from build123d import *

# Parameters (mm, degrees)
SKETCH1_R           = 2.5
BOSS_EXTRUDE1_DEPTH = 30
SKETCH6_R           = 3.75
BOSS_EXTRUDE6_DEPTH = 15
BOSS_EXTRUDE2_DEPTH = 2.5
SKETCH3_R           = 2.5
BOSS_EXTRUDE3_DEPTH = 2.8
BOSS_EXTRUDE4_START = 2.8
BOSS_EXTRUDE4_DEPTH = 2.8
SKETCH5_R           = 2.5
BOSS_EXTRUDE5_DEPTH = 2.8


with BuildPart() as part:
    # Sketch1 → Boss-Extrude1 (new, symmetric)
    with BuildSketch(Plane(origin=(0, 0, 0), x_dir=(1, 0, 0), z_dir=(0, 1, 0))):
        with Locations(Location((0, 0, 0), (0, 0, 270))):
            Circle(SKETCH1_R)
    extrude(amount=BOSS_EXTRUDE1_DEPTH, both=True)

    # Sketch6 → Boss-Extrude6 (add, symmetric)
    with BuildSketch(Plane(origin=(0, 0, 0), x_dir=(1, 0, 0), z_dir=(0, 1, 0))):
        with Locations(Location((0, 0, 0), (0, 0, 270))):
            Circle(SKETCH6_R)
    extrude(amount=BOSS_EXTRUDE6_DEPTH, both=True)

    # Sketch2 → Boss-Extrude2 (add)
    with BuildSketch(Plane(origin=(0, 30, 0), x_dir=(1, 0, 0), z_dir=(0, 1, 0))):
        with BuildLine():
            Line((0, 5), (12.5, 5))
            ThreePointArc((12.5, 5), (17.5, 0), (12.5, -5))
            Line((12.5, -5), (0, -5))
            ThreePointArc((0, -5), (-5, 0), (0, 5))
        make_face()
    extrude(amount=BOSS_EXTRUDE2_DEPTH)

    # Sketch3 → Boss-Extrude3 (add)
    with BuildSketch(Plane(origin=(0, 32.5, 0), x_dir=(1, 0, 0), z_dir=(0, 1, 0))):
        with Locations(Location((12.5, 0, 0), (0, 0, 270))):
            Circle(SKETCH3_R)
    extrude(amount=BOSS_EXTRUDE3_DEPTH)

    # Sketch4 → Boss-Extrude4 (add)
    with BuildSketch(Plane.XZ.offset(30).offset(BOSS_EXTRUDE4_START)):
        with BuildLine():
            Line((0, -5), (-12.5, -5))
            ThreePointArc((-12.5, -5), (-17.5, 0), (-12.5, 5))
            Line((-12.5, 5), (0, 5))
            ThreePointArc((0, 5), (5, 0), (0, -5))
        make_face()
    extrude(amount=-BOSS_EXTRUDE4_DEPTH)

    # Sketch5 → Boss-Extrude5 (add)
    with BuildSketch(Plane.XZ.offset(32.8)):
        with Locations(Location((-12.5, 0, 0), (0, 0, 270))):
            Circle(SKETCH5_R)
    extrude(amount=BOSS_EXTRUDE5_DEPTH)


solid = part.part
The model under review builds one solid part; all positions refer to its coordinate system, in mm. A direction names the side the tool comes from. Coordinates: 2 decimals unless noted, no trailing zeros. Write each loop counter-clockwise with the first axis right and the second up, starting at its lowest first coordinate (ties: lowest second). Pieces come first, ordered by that corner, then holes. Notation, with made-up numbers: M 54.5,24 L 107.5,24 A27 ccw 107.5,49 Z; hole C 8.5,8.25 d7. An arc over 180 degrees is marked long. Put each result on its own line as item: value.
1) Draft analysis for pull direction Y (two halves, no side actions). For faces 5 (the cylindrical face through (17.5, 31.2, -0.1)), 6 (the cylindrical face through (-2.44, -22.4, -0.54)), 7 (the flat face through (3, 15, 0)), 8 (the flat face through (6, 32.5, 0)), state which applies: released by +Y, released by -Y, zero draft, split by the parting line, or undercut.
Computed:
face 5: zero draft
face 6: undercut
face 7: undercut
face 8: released by +Y
2) Wall thickness on probe 1 along Y at (x, z) = (2, 2.75); probe 2 along Y at (x, z) = (-3, 3.5); probe 3 along X at (y, z) = (-13, -0.25): over which ranges is each line inside the solid? List them lowest first. Write a range as [from, to].
Computed:
probe 1: y = [-32.8, -30], [-15, 15], [30, 32.5]
probe 2: y = [-32.8, -30], [30, 32.5]
probe 3: x = [-3.74, 3.74]
3) Add section C-C on y = -21.5. Give the boundary of the cut face in (x, z), then the cut area to 3 significant figures.
Computed:
outline: C 0,0 d5
area: 19.6 mm2
4) For faces 1 (the cylindrical face through (-2.44, 22.6, -0.54)), 2 (the cylindrical face through (-5, 31, 0)), 3 (the cylindrical face through (10.06, 33.88, -0.54)), 4 (the cylindrical face through (5, -31, 0)), list the 3-axis set-ups (+Z, -Z, +X, -X, +Y, -Y) from which the entire face can be reached by the end or side of a thin tool; tool diameter is ignored.
Computed:
face 1: none
face 2: -X, +Y
face 3: +Y
face 4: +X, -Y
5) Clearance check with flat-ended pins moving along their axes: pin 1 Ø6 at (x, z) = (1.5, -1.5) entering from -Y; pin 2 Ø8 at (x, y) = (-8.5, -19) entering from +Z; pin 3 Ø1 at (y, z) = (-1.5, 1) entering from +X; pin 4 Ø1.5 at (y, z) = (-26, 0) entering from +X. State where each tip first meets the part, or that it passes through.
Computed:
pin 1: stops at y = -32.8
pin 2: passes through
pin 3: stops at x = 3.72
pin 4: stops at x = 2.5
6) Add section B-B on x = -8. Give the boundary of the cut face in (y, z), then the cut area to 3 significant figures.
Computed:
outline: M -32.8,-5 L -30,-5 L -30,5 L -32.8,5 Z
area: 28.0 mm2
7) Add section A-A on y = 0. Give the boundary of the cut face in (x, z).
Computed:
outline: C 0,0 d7.5
